Autodesk Inventor part; units mm, degrees
ref_plane "YZ Plane" through (0, 0, 0) normal (1, 0, 0) x (0, 1, 0)
ref_plane "XY Plane" through (0, 0, 0) normal (0, 0, 1) x (1, 0, 0)
sketch "Sketch1" plane through (0, 0, 0) normal (0, 0, 1) x (1, 0, 0)
  arc A0 (20.833333, 123.251662) -> (-20.833333, 123.251662) centre (0, 0) ccw
  arc A1 (20, 118.321596) -> (-20, 118.321596) centre (0, 0) ccw
  line L0 (-20, 118.321596) -> (-20.833333, 123.251662)
  line L1 (0, 0) -> (0, 133.48158) construction
  line L2 (20, 118.321596) -> (20.833333, 123.251662)
  dimension "d0" = 250
  dimension "d1" = 5
  dimension "d2" = 40
extrude "Extrusion1" add sketch "Sketch1" along normal mid plane 40
ref_plane "Work Plane3" through (0, 87, 0) normal (0, 1, 0) x (-1, 0, 0)
ref_plane "Work Plane2" through (0, 125, 0) normal (0, 1, 0) x (-1, 0, 0)
sketch "Sketch3" plane through (0, 87, 0) normal (0, 1, 0) x (-1, 0, 0)
  line L0 (10, -10) -> (-10, -10)
  line L1 (-10, -10) -> (-10, 10)
  line L2 (-10, 10) -> (10, 10)
  line L3 (10, 10) -> (10, -10)
  line L4 (10, -10) -> (-10, 10) construction
  line L5 (-10, -10) -> (10, 10) construction
  point P0 (0, 0)
  dimension "d6" = 20
  dimension "d7" = 20
extrude "Extrusion2" add sketch "Sketch3" along normal up to next
sketch "Sketch4" plane through (0, 125, 0) normal (0, 1, 0) x (-1, 0, 0)
  circle A0 centre (0, 0) radius 5.3
  dimension "d10" = 10.6
extrude "Extrusion3" cut sketch "Sketch4" against normal blind 34
properties part number "shiftt_fixed_plate" material "Acetal Resin, Black"
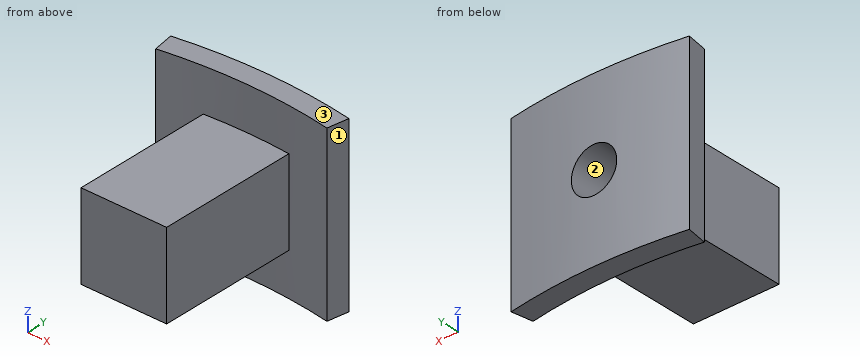
Here's how the part is built. I have some questions about the finished solid (model axes, mm). Face numbers are marked on the shaded views. Round coordinates to 2 decimals unless told otherwise and drop trailing zeros. Loops run counter-clockwise (first coordinate to the right, second up) from the corner with the lowest first, then second, coordinate; pieces in that order, holes last. Notation, with made-up numbers: M -13,-29 L 8,-29 A14 cw 8,-7 Z; hole C 89,8.25 d9. An arc over 180 degrees is marked long. Write each question's results on one line, items separated by ' | '. Start each with the question number.
(1) I want a section at C-C (z = -2). Please give me the cut outline in (x, y), then the cut area to 3 significant figures.
(2) I want a section at D-D (x = 9). Please give me the cut outline in (y, z).
(3) I want a section at A-A (y = 96.5). Please give me the cut outline in (x, z).
(4) I want a section at B-B (x = 0). Please give me the cut outline in (y, z), then the cut area to 3 significant figures.
(5) Will these pins go through, and if not, where does the flat tip stop? P1, Ø6, axis at x = 4, y = 103.5, coming from the +Z side; P2, Ø10, axis at y = 117.5, z = 8, coming from the -X side; P3, Ø12, axis at y = 94.5, z = -14.5, coming from the -X side.
(6) Thinking about a two-plate mould opening in X: for the marked faces 1, 2 and 3, which applies, pulls with the +X half, pulls with the -X half, needs draft (parallel to the pull), parting line crosses it, or undercut?
(7) If I drill on probe 1 along Z at (x, y) = (0, 112); probe 2 along Y at (x, z) = (-0.5, 7.5), over which ranges is the centre line in solid material (lowest first)? Write a range as from..to.
Solved:
1) outline: M -20.83,123.25 L -20,118.32 A120 cw -10,119.58 L -10,87 L 10,87 L 10,119.58 A120 cw 20,118.32 L 20.83,123.25 A125 ccw 4.91,124.9 L 4.91,91 L -4.91,91 L -4.91,124.9 A125 ccw Z | area: 529 mm²
2) outline: M 87,-10 L 119.66,-10 L 119.66,-20 L 124.68,-20 L 124.68,20 L 119.66,20 L 119.66,10 L 87,10 Z
3) outline: M -10,-10 L 10,-10 L 10,10 L -10,10 Z; hole C 0,0 d10.6
4) outline: M 87,-10 L 120,-10 L 120,-20 L 125,-20 L 125,-5.3 L 91,-5.3 L 91,5.3 L 125,5.3 L 125,20 L 120,20 L 120,10 L 87,10 Z | area: 500 mm²
5) P1: stops at z = 10 | P2: stops at x = -20.71 | P3: stops at x = -10
6) face 1: pulls with the +X half | face 2: undercut | face 3: needs draft
7) probe 1: z = -10..-5.3, 5.3..10 | probe 2: y = 87..125
